Source: three-view drawing plus pictorial views. Frame: mm from the lowest corner of the part. A direction names the side the tool comes from. Give positions to 0.01 mm unless a question says otherwise; leave off trailing zeros. Order: outer loops, then holes, each group sorted by start corner. A loop starts at its lowest first (then second) coordinate and runs counter-clockwise, first axis right, second up. Notation, with made-up numbers: (64.25, 11.25) -> (114.25, 11.25) arc R25 ccw to (114.25, 24.25) -> close; hole circle Ø8 at (80.5, 40). An arc over 180 degrees is marked (long way). Answer in a Markdown table with one row per item. Add a question column.
Q1. Set-up query: the marked faces 1 and 2. Return all of +Z, -Z, +X, -X, +Y, -Y with unobstructed straight access to the full face (end or side cutting, diameter ignored); none if empty.
Q2. Cut plane B-B on x = 16. Return the cut outline in (y, z).
Q3. Cut plane A-A on y = 9.25. Return the cut outline in (x, z) (1 decimal).
Q4. Pull-direction query (X, two-part tool) for the marked faces 3 and 4; classes: +X half, -X half, draft (parallel to the pull), parting line (faces both ways), or undercut.
Q5. Contact query for flat-ended pins moving along their axis: P1, Ø3, axis at y = 7, z = 16.5, coming from the -X side; P2, Ø3, axis at y = 8.5, z = 23.5, coming from the +X side (1 decimal); P3, Ø1.3, axis at y = 5, z = 11.5, coming from the -X side. Output: stop coordinate, or through.
Q6. Cut plane D-D on z = 26. Return the cut outline in (x, y) (1 decimal).
Q7. Line query: line 1 along Z through (x, y) = (12, 5) (1 decimal); line 2 along X through (y, z) = (4.25, 14.75) (1 decimal); line 3 along Z through (x, y) = (24.25, 5) (1 decimal). Output: solid intervals per line, ascending. Write a range as from..to.
Q8. Cut plane C-C on z = 10. Return the cut outline in (x, y).
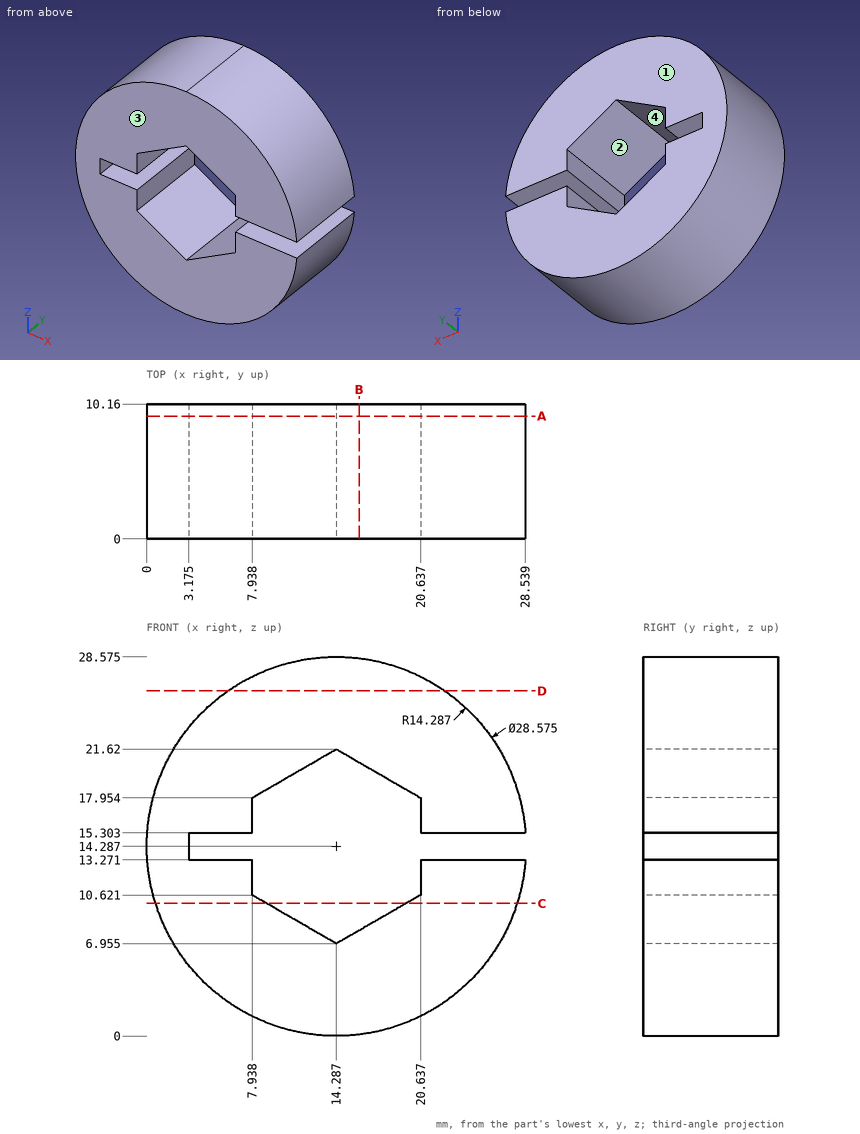
Completed:
| question | item | result |
|---|---|---|
| 1 | face 1 | +Z, -Z, +X, -X, +Y |
| 1 | face 2 | +Y, -Y |
| 2 | outline | (0, 0.1) -> (10.16, 0.1) -> (10.16, 7.94) -> (0, 7.94) -> close; (0, 20.63) -> (10.16, 20.63) -> (10.16, 28.47) -> (0, 28.47) -> close |
| 3 | outline | (3.2, 13.3) -> (3.2, 15.3) -> (7.9, 15.3) -> (7.9, 18) -> (14.3, 21.6) -> (20.6, 18) -> (20.6, 15.3) -> (28.5, 15.3) arc R14.3 ccw (long way) to (28.5, 13.3) -> (20.6, 13.3) -> (20.6, 10.6) -> (14.3, 7) -> (7.9, 10.6) -> (7.9, 13.3) -> close |
| 4 | face 3 | draft |
| 4 | face 4 | undercut |
| 5 | P1 | stops at x = 0.02 |
| 5 | P2 | stops at x = 26.3 |
| 5 | P3 | stops at x = 0.16 |
| 6 | outline | (6.1, 0) -> (22.5, 0) -> (22.5, 10.2) -> (6.1, 10.2) -> close |
| 7 | line 1 | z = 0.2..8.3, 20.3..28.4 |
| 7 | line 2 | x = 0..3.2 |
| 7 | line 3 | z = 4..13.3, 15.3..24.5 |
| 8 | outline | (0.66, 0) -> (9.01, 0) -> (9.01, 10.16) -> (0.66, 10.16) -> close; (19.56, 0) -> (27.92, 0) -> (27.92, 10.16) -> (19.56, 10.16) -> close |
